from build123d import *

# Parameters (mm, degrees)
SKETCH012_W             = 16
SKETCH012_H             = 16
PAD001_DEPTH            = 4
POCKET011_DEPTH         = 16.001
POCKET012_DEPTH         = 16.001
SKETCH015_W             = 2.9
SKETCH015_H             = 6.9
PAD002_DEPTH            = 2.5
CHAMFER_SIZE            = 0.5
BODY002_PLACEMENT_ANGLE = 180


with BuildPart() as part:
    # Sketch012 (on XY_Plane002 of Origin004) → Pad001 (new body)
    with BuildSketch(Plane.XY):
        with Locations((130.823461, 8)):
            Rectangle(SKETCH012_W, SKETCH012_H)
    extrude(amount=PAD001_DEPTH)

    # Sketch013 (on Face1 of Pad001) → Pocket011 (cut, through all)
    with BuildSketch(Plane.XZ):
        with BuildLine():
            ThreePointArc((123.723461, 4), (123.051239, 2.05), (122.823461, 0))
            Line((122.823461, 4), (122.823461, 0))
            Line((123.723461, 4), (122.823461, 4))
        make_face()
        with BuildLine():
            ThreePointArc((138.823461, 0), (138.595683, 2.05), (137.923461, 4))
            Line((137.923461, 4), (138.823461, 4))
            Line((138.823461, 4), (138.823461, 0))
        make_face()
    extrude(amount=-POCKET011_DEPTH, mode=Mode.SUBTRACT)

    # Sketch014 (on Face2 of Pad001) → Pocket012 (cut, through all)
    with BuildSketch(Plane.YZ.offset(138.823461)):
        with BuildLine():
            ThreePointArc((0.5, 4), (0.125485, 2.015564), (0, 0))
            Line((0, 0), (0, 4))
            Line((0.5, 4), (0, 4))
        make_face()
        with BuildLine():
            ThreePointArc((16, 0), (15.874515, 2.015564), (15.5, 4))
            Line((15.5, 4), (16, 4))
            Line((16, 4), (16, 0))
        make_face()
    extrude(amount=-POCKET012_DEPTH, mode=Mode.SUBTRACT)

    # Sketch015 → Pad002 (join)
    with BuildSketch(Plane(origin=(127.960214, 8.35, 0), x_dir=(0, 1, 0), z_dir=(0, 0, -1))):
        with Locations((-0.35, 2.863247)):
            Rectangle(SKETCH015_W, SKETCH015_H)
    extrude(amount=PAD002_DEPTH)

    # Chamfer
    chamfer_edges = [part.edges().sort_by_distance(p)[0] for p in [
        (123.054343, 0.131581, 2.06375),
        (138.592578, 0.131581, 2.06375),
        (138.592578, 15.868419, 2.06375),
        (123.054343, 15.868419, 2.06375),
        (123.723461, 8, 4),
        (130.823461, 15.5, 4),
        (137.923461, 8, 4),
        (130.823461, 0.5, 4),
    ]]
    chamfer(chamfer_edges, length=CHAMFER_SIZE)


with BuildPart() as part_1:
    # Body002 placement: moved
    add(part.part.moved(Location((48.422, -12.144, 0))).rotate(Axis((48.422, -12.144, 0), (1, 0, 0)), BODY002_PLACEMENT_ANGLE))


solid = part_1.part
Geometry: final body of the model. Coordinates: model frame, mm. A direction names the side the tool comes from. Coordinates: 2 decimals unless noted, no trailing zeros. Loops run counter-clockwise (first coordinate to the right, second up) from the corner with the lowest first, then second, coordinate; pieces in that order, holes last. Notation, with made-up numbers: (-8.5, 30.25) - (21.5, 30.25) arc R22 ccw to (21.5, 59.25) - close; hole circle Ø4 at (37, 12). An arc over 180 degrees is marked (long way). Put each result on its own line as item: value. Start each with the question number.
Q1. Cut plane D-D, the plane x = 180.5. Return loops of the section in (y, z), and give its area (3 significant figures).
Q2. Cut plane A-A, the plane x = 184.25. Return loops of the section in (y, z).
Q3. Set-up query: faces 1 (the cylindrical face through (179.35, -28.05, -1.74)), 2 (the flat face through (179, -21.594, 1)), 3 (the flat face through (182.695, -20, 1)), 4 (the flat face through (175.795, -20, 1)), 5 (the flat face through (179, -18.694, 1)). Return all of +Z, -Z, +X, -X, +Y, -Y with unobstructed straight access to the full face (end or side cutting, diameter ignored); none if empty.
Q4. Pin query (flat end, axial travel): pin 1 Ø1.5 at (y, z) = (-20, -2) entering from +X; pin 2 Ø2 at (x, z) = (179.5, 1.5) entering from -Y; pin 3 Ø1.3 at (y, z) = (-20.5, 1.5) entering from +X. Return the tip coordinate at first contact, or that it passes through.
Q5. Line query: line 1 (Z direction, x = 174.75, y = -17); line 2 (Y direction, x = 182.75, z = -3.5); line 3 (Y direction, x = 176, z = -0.25). Output: solid intervals per line, ascending.
Q6. Cut plane B-B, the plane y = -25.5. Return loops of the section in (x, z).
Q7. Cut plane C-C, the plane z = 1.5. Return loops of the section in (x, y).
Filled sheet:
1. outline: (-28.14, 0) arc R16.25 ccw to (-27.76, -3.51) - (-27.14, -4) - (-13.14, -4) - (-12.53, -3.51) arc R16.25 ccw to (-12.14, 0) - (-18.69, 0) - (-18.69, 2.5) - (-21.59, 2.5) - (-21.59, 0) - close
1. area: 69.7 mm²
2. outline: (-28.14, 0) arc R16.25 ccw to (-27.76, -3.51) - (-27.14, -4) - (-13.14, -4) - (-12.53, -3.51) arc R16.25 ccw to (-12.14, 0) - close
3. face 1: -Z, +X, -X, -Y
3. face 2: +Z, +X, -X, -Y
3. face 3: +Z, +X, +Y, -Y
3. face 4: +Z, -X, +Y, -Y
3. face 5: +Z, +X, -X, +Y
4. pin 1: x = 187.16
4. pin 2: y = -21.59
4. pin 3: x = 182.7
5. line 1: -4 to 0
5. line 2: -27.76 to -12.53
5. line 3: -28.14 to -12.15
6. outline: (171.25, 0) arc R9.34 ccw to (171.94, -3.54) - (172.65, -4) - (185.85, -4) - (186.55, -3.54) arc R9.34 ccw to (187.25, 0) - close
7. outline: (175.8, -21.59) - (182.7, -21.59) - (182.7, -18.69) - (175.8, -18.69) - close
